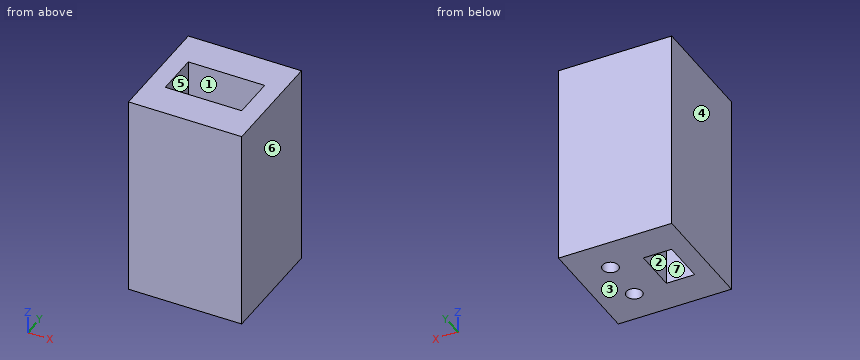
```python
from build123d import *

# Parameters (mm, degrees)
F0_W     = 20
F0_H     = 20
F0_W_2   = 13.5
F0_H_2   = 7.7
F1_DEPTH = 26
F2_W     = 20
F2_H     = 20
F2_W_2   = 5
F2_H_2   = 7.7
F3_DEPTH = 10
F4_R     = 1.4
F5_DEPTH = 10


with BuildPart() as f1:
    # F0 (on Top) → F1 (new body)
    with BuildSketch(Plane.XY):
        Rectangle(F0_W, F0_H)
        Rectangle(F0_W_2, F0_H_2, mode=Mode.SUBTRACT)
    extrude(amount=F1_DEPTH)

    # F2 (on Top) → F3 (join)
    with BuildSketch(Plane.XY):
        Rectangle(F2_W, F2_H)
        with Locations((-4.25, 0)):
            Rectangle(F2_W_2, F2_H_2, mode=Mode.SUBTRACT)
    extrude(amount=-F3_DEPTH)

    # F4 (on face) → F5 (cut)
    with BuildSketch(Plane(origin=(0, 0, -10), x_dir=(1, 0, 0), z_dir=(0, 0, -1))):
        with Locations((4, 4)):
            Circle(F4_R)
        with Locations((4, -4)):
            Circle(F4_R)
    extrude(amount=-F5_DEPTH, mode=Mode.SUBTRACT)


solid = f1.part
```
Check sheet for the modelled part. Datum: model origin and axes. Units: mm. Face numbers are marked on the shaded views. A direction names the side the tool comes from. Round coordinates to 2 decimals unless told otherwise and drop trailing zeros. Write each loop counter-clockwise with the first axis right and the second up, starting at its lowest first coordinate (ties: lowest second). Pieces come first, ordered by that corner, then holes. Notation, with made-up numbers: M 5.5,71 L 9.5,71 A23 cw 9.5,94 Z; hole C 29.5,-3.75 d6. An arc over 180 degrees is marked long. Write item = value, one per line. Start each with the question number.
1. Gauge pin test, flat ends, axial feed: pin 1 (4 mm diameter, centred on x = 3.5, y = 1, fed in from +Z); pin 2 (0.5 mm diameter, centred on x = 3.5, y = 4.5, fed in from -Z). Record the tip position at first contact, or that the pin passes through.
2. Scan lines: line 1 (Y direction, x = 4, z = -7.25); line 2 (Y direction, x = 3.5, z = 8); line 3 (X direction, y = 4, z = -2.5). Record each from-to range of solid material in increasing order. Write a range as [from, to].
3. Section check A-A, the plane x = -6. Record the cut outline in (y, z), then the cut area to 3 significant figures.
4. Section check D-D, the plane z = -1. Record the cut outline in (x, y).
5. Release check for a two-part mould opening along X. For the marked faces 1, 2, 3 and 4 record: pulls with the +X half, pulls with the -X half, needs draft (parallel to the pull), parting line crosses it, or undercut.
6. Section check C-C, the plane x = 4. Record the cut outline in (y, z).
7. Section check B-B, the plane z = 9. Record the cut outline in (x, y).
8. Tool access check on the marked faces 5, 6 and 7. Record the directions out of +Z, -Z, +X, -X, +Y, -Y that give a thin tool (end or side, any length) a straight path to the whole face; none if there is none.
Results found:
q1.pin_1 = 0
q1.pin_2 = 0
q2.line_1 = [-10, -5.4], [-2.6, 2.6], [5.4, 10]
q2.line_2 = [-10, -3.85], [3.85, 10]
q2.line_3 = [-10, 2.6], [5.4, 10]
q3.outline = M -10,-10 L -3.85,-10 L -3.85,26 L -10,26 Z; M 3.85,-10 L 10,-10 L 10,26 L 3.85,26 Z
q3.area = 443 mm^2
q4.outline = M -10,-10 L 10,-10 L 10,10 L -10,10 Z; hole M -6.75,-3.85 L -1.75,-3.85 L -1.75,3.85 L -6.75,3.85 Z; hole C 4,-4 d2.8; hole C 4,4 d2.8
q5.face_1 = undercut
q5.face_2 = undercut
q5.face_3 = needs draft
q5.face_4 = pulls with the -X half
q6.outline = M -10,-10 L -5.4,-10 L -5.4,0 L -3.85,0 L -3.85,26 L -10,26 Z; M -2.6,-10 L 2.6,-10 L 2.6,0 L -2.6,0 Z; M 3.85,0 L 5.4,0 L 5.4,-10 L 10,-10 L 10,26 L 3.85,26 Z
q7.outline = M -10,-10 L 10,-10 L 10,10 L -10,10 Z; hole M -6.75,-3.85 L 6.75,-3.85 L 6.75,3.85 L -6.75,3.85 Z
q8.face_5 = +Z, -Z
q8.face_6 = +Z, -Z, +X, +Y, -Y
q8.face_7 = +Z
